```python
from build123d import *

# Parameters (mm, degrees)
F1_DEPTH = 7.7
F2_R     = 2
F3_DEPTH = 14.4


with BuildPart() as f1:
    # F0 (on Top) → F1 (new body)
    with BuildSketch(Plane.XY):
        Polygon((-38.868088, 39.890725), (-37.658811, 39.446436), (-38.249725, 38.189034), (-38.750622, 36.540247), (-38.750622, 34.333538), (-39.874792, 32.168467), (-40.947256, 29.788468), (-41.671675, 27.403923), (-42.248044, 25.506711), (-42.248044, 23.882907), (-43.663666, 22.30031), (-44.865134, 20.796624), (-46.453279, 20.09597), (-12.089583, 20.09597), (-12.089583, 20.809148), (-12.285668, 21.436621), (-12.285668, 22.30031), (-12.727885, 23.013672), (-12.727885, 23.801431), (-12.727885, 24.664005), (-12.727885, 25.523571), (-12.528915, 26.178513), (-12.476629, 26.770333), (-12.320494, 27.284278), (-12.248813, 27.708853), (-12.088908, 28.056234), (-11.851807, 28.475296), (-11.526482, 29.291363), (-11.383266, 30.11846), (-11.383266, 30.81312), (-11.926459, 32.551334), (-12.7981, 34.52705), (-13.276388, 36.057569), (-13.579202, 37.026573), (-13.276388, 39.824102), (-13.276388, 41.953199), (-12.412329, 43.710936), (-11.989028, 45.443922), (-11.394863, 47.399715), (-10.874968, 48.711833), (-10.280802, 49.825892), (-9.63011, 50.777867), (-7.760718, 52.413587), (-7.153935, 53.932466), (-7.153935, 55.135302), (-7.64388, 56.245841), (-8.157964, 56.853395), (-9.022558, 57.507679), (-9.583375, 57.046662), (-10.421853, 57.046662), (-11.4294, 57.484314), (-11.703454, 56.853395), (-11.703454, 56.161334), (-12.412329, 55.848595), (-12.412329, 57.554416), (-12.412329, 58.947231), (-12.714608, 59.914522), (-13.579202, 61.12963), (-14.490531, 62.274631), (-15.799105, 63.278936), (-16.500128, 62.57841), (-17.317986, 61.620343), (-18.248623, 60.544401), (-18.991331, 59.603639), (-19.808309, 58.539093), (-20.58815, 57.610705), (-21.566048, 56.558538), (-22.333512, 55.704426), (-23.076219, 54.899827), (-23.905577, 54.045714), (-24.474986, 53.587709), (-25.415219, 52.8854), (-26.653593, 52.498408), (-28.460847, 52.127052), (-30.104453, 51.151142), (-30.863894, 50.566956), (-31.407185, 50.064556), (-31.921268, 49.597207), (-32.581396, 49.013022), (-33.083797, 48.516467), (-33.60372, 48.019908), (-34.222957, 47.52335), (-35.035051, 46.96336), (-35.73864, 46.594702), (-36.679402, 46.241917), (-38.461901, 45.684885), (-39.5265, 45.352735), (-40.787674, 44.796333), (-41.770652, 44.239931), (-42.577434, 43.525882), (-43.022554, 42.867474), (-42.790722, 42.255431), (-41.640826, 41.328095), (-40.19418, 40.549133), align=None)
    extrude(amount=F1_DEPTH)

    # F2 (on face) → F3 (cut)
    with BuildSketch(Plane.XY.offset(7.7)):
        with Locations((-27.663102, 49.291145)):
            Circle(F2_R)
    extrude(amount=-F3_DEPTH, mode=Mode.SUBTRACT)


solid = f1.part
```
Work out the finished part from the listing and answer in its coordinate system (mm). A direction names the side the tool comes from. Coordinates: 2 decimals unless noted, no trailing zeros. Loops run counter-clockwise (first coordinate to the right, second up) from the corner with the lowest first, then second, coordinate; pieces in that order, holes last.
1) Flat-ended cylindrical pins translate along their axes: pin 1 (1.3 mm diameter, centred on y = 24.5, z = 2, fed in from -X); pin 2 (0.7 mm diameter, centred on y = 35, z = 3.5, fed in from -X); pin 3 (1 mm diameter, centred on y = 48, z = 7, fed in from +X). Find the tip coordinate at first contact, or state that the pin passes through.
Results:
pin 1: stops at x = -42.28
pin 2: stops at x = -38.75
pin 3: stops at x = -10.96
2) For faces 4 (the flat face through (-11.65, 31.67, 3.8)), 5 (the flat face through (-36.2, 46.42, 3.8)), 6 (the flat face through (-40.928, 40.944, 3.796)), determine the directions among +Z, -Z, +X, -X, +Y, -Y from which every point of the face is accessible in a straight line to the end or side of a thin tool.
Results:
face 4: +Z, -Z, +X
face 5: +Z, -Z, -X, +Y
face 6: +Z, -Z, -X
3) Consider probe 1 along X at (y, z) = (25, 5.5); probe 2 along Y at (x, z) = (-38, 7); probe 3 along Y at (x, z) = (-29.5, 6.5). Determine where each line is inside the solid, lowest interval first.
Results:
probe 1: x = -42.25 to -12.73
probe 2: y = 20.1 to 38.72, 39.57 to 45.83
probe 3: y = 20.1 to 48.5, 50.08 to 51.51
4) For a pull along Y with two mould halves and no side action, classify faces 1 (the flat face through (-26.026, 52.695, 3.796)), 2 (the flat face through (-42.95, 23.1, 3.8)), 3 (the flat face through (-7.154, 54.5, 3.8)) as +Y half, -Y half, draft (parallel to the pull), parting line (faces both ways), or undercut.
Results:
face 1: +Y half
face 2: undercut
face 3: draft
5) Section A-A (y = 31.5) is taken. Give the vertices of the cut face in (x, z), plus the area to 3 significant figures.
Results:
outline: (-40.18, 0) - (-11.6, 0) - (-11.6, 7.7) - (-40.18, 7.7) - close
area: 220 mm2
